Print and shaded views of the part. All mm, measured from the part's lowest x, y and z. A direction names the side the tool comes from. Coordinates: 2 decimals unless noted, no trailing zeros. Order: outer loops, then holes, each group sorted by start corner. A loop starts at its lowest first (then second) coordinate and runs counter-clockwise, first axis right, second up. Notation, with made-up numbers: (22, 51) -> (27, 51) arc R20 cw to (27, 85) -> close; hole circle Ø6 at (55, -19.75). An arc over 180 degrees is marked (long way). Write item = value, one per line. Start each with the question number.
Q1. Flat gauge pins, fed straight in: pin 1 (3 mm diameter, centred on y = 6.5, z = 3, fed in from -X); pin 2 (4 mm diameter, centred on y = 9.5, z = 7.5, fed in from +X); pin 3 (0.8 mm diameter, centred on x = 13.5, z = 8.5, fed in from +Y). Where does each tip first touch, or does it go through?
Q2. Mould opens along Z. For the marked faces 1, 2 and 3 say: +Z half, -Z half, draft (parallel to the pull), parting line (faces both ways), or undercut.
Q3. Cut at C-C, the plane z = 3.75. List the corners of the cut face in (x, y) (1 decimal).
Q4. Wall check: line 1 (Y direction, x = 16.25, z = 5.5) (1 decimal); line 2 (Y direction, x = 13.5, z = 1.5); line 3 (Z direction, x = 4.25, y = 7). Give the ranges that are in metal, low to high. Write a range as from..to.
Q5. 3-axis set-ups, long thin cutter, end or side, ignore diameter. For the marked faces 4 and 5: which of +Z, -Z, +X, -X, +Y, -Y reach the whole face in a straight line?
Q6. Cut at A-A, the plane y = 13.98. List the corners of the cut face in (x, z) (1 decimal).
Q7. Cut at D-D, the plane x = 4. List the corners of the cut face in (y, z) (1 decimal).
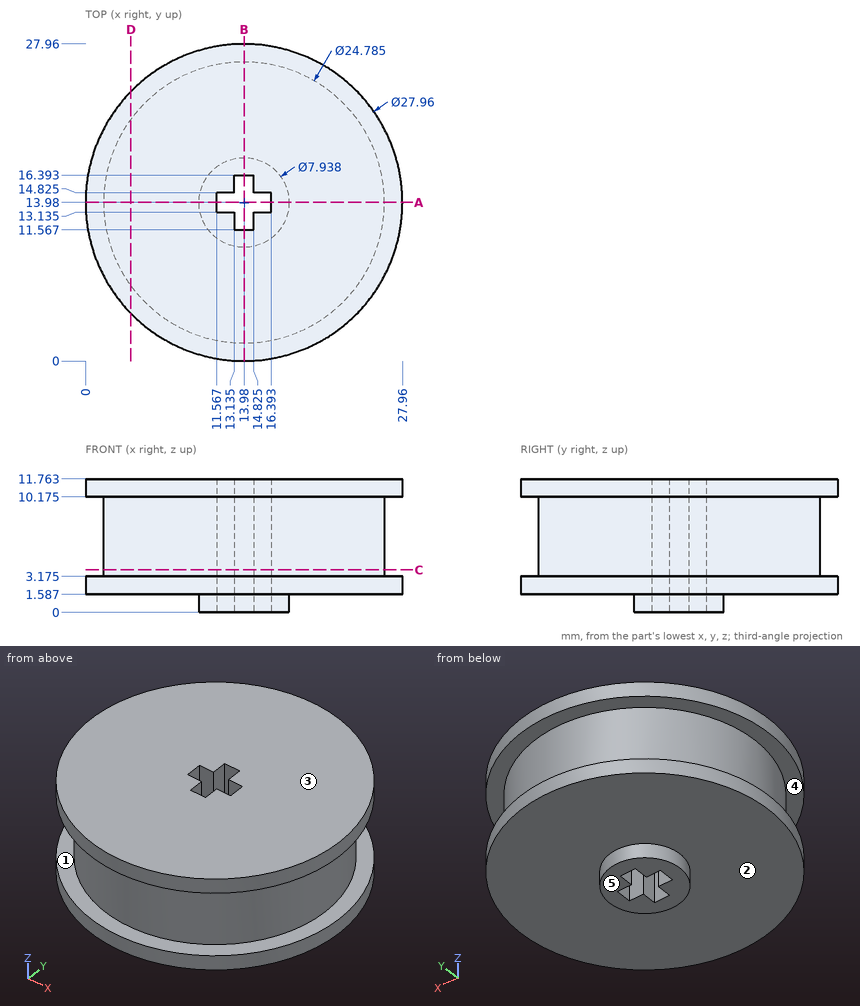
Here are the results:
q1.pin_1 = 1.34
q1.pin_2 = 26.12
q1.pin_3 = 26.37
q2.face_1 = undercut
q2.face_2 = -Z half
q2.face_3 = +Z half
q3.outline = circle Ø24.8 at (14, 14); hole (11.6, 13.1) -> (13.1, 13.1) -> (13.1, 11.6) -> (14.8, 11.6) -> (14.8, 13.1) -> (16.4, 13.1) -> (16.4, 14.8) -> (14.8, 14.8) -> (14.8, 16.4) -> (13.1, 16.4) -> (13.1, 14.8) -> (11.6, 14.8) -> close
q4.line_1 = 1.8..13.1, 14.8..26.2
q4.line_2 = 10.04..11.57, 16.39..17.92
q4.line_3 = 1.59..11.76
q5.face_4 = none
q5.face_5 = -Z, +X, -X, +Y, -Y
q6.outline = (0, 1.6) -> (10, 1.6) -> (10, 0) -> (11.6, 0) -> (11.6, 11.8) -> (0, 11.8) -> (0, 10.2) -> (1.6, 10.2) -> (1.6, 3.2) -> (0, 3.2) -> close; (16.4, 0) -> (17.9, 0) -> (17.9, 1.6) -> (28, 1.6) -> (28, 3.2) -> (26.4, 3.2) -> (26.4, 10.2) -> (28, 10.2) -> (28, 11.8) -> (16.4, 11.8) -> close
q7.outline = (4.2, 1.6) -> (23.8, 1.6) -> (23.8, 3.2) -> (21.3, 3.2) -> (21.3, 10.2) -> (23.8, 10.2) -> (23.8, 11.8) -> (4.2, 11.8) -> (4.2, 10.2) -> (6.6, 10.2) -> (6.6, 3.2) -> (4.2, 3.2) -> close
